The model under review builds one solid part; all positions refer to its coordinate system, in mm. A direction names the side the tool comes from. Give positions to 0.01 mm unless a question says otherwise; leave off trailing zeros. Order: outer loops, then holes, each group sorted by start corner. A loop starts at its lowest first (then second) coordinate and runs counter-clockwise, first axis right, second up.
```python
from build123d import *

# Parameters (mm, degrees)
SKETCH1_W               = 27
SKETCH1_H               = 129
BOSS_EXTRUDE1_DEPTH     = 1.5
FILLET1_R               = 3
SKETCH3_W               = 6
SKETCH3_H               = 3
CUT_EXTRUDE2_DEPTH      = 2.5
CUT_EXTRUDE2_DEPTH_BACK = 2.5
CUT_EXTRUDE4_DEPTH      = 2.5
CUT_EXTRUDE4_DEPTH_BACK = 2.5
FILLET2_R               = 3
FILLET2_2_R             = 1.5
CUT_EXTRUDE3_DEPTH      = 5
SKETCH2_W               = 3
SKETCH2_H               = 35
CUT_EXTRUDE1_DEPTH      = 2.5000001
CUT_EXTRUDE1_DEPTH_BACK = 2.5000001


with BuildPart() as part:
    # Sketch1 → Boss-Extrude1 (new body, symmetric)
    with BuildSketch(Plane(origin=(0, 0, 0), x_dir=(1, 0, 0), z_dir=(0, 1, 0))):
        Rectangle(SKETCH1_W, SKETCH1_H)
    extrude(amount=BOSS_EXTRUDE1_DEPTH, both=True)

    # Fillet1
    fillet1_edges = [part.edges().sort_by_distance(p)[0] for p in [
        (-13.5, 0, -64.5),
        (13.5, 0, -64.5),
    ]]
    fillet(fillet1_edges, radius=FILLET1_R)

    # Sketch3 → Cut-Extrude2 (cut, two sides)
    with BuildSketch(Plane(origin=(0, 0, 0), x_dir=(1, 0, 0), z_dir=(0, 1, 0))) as cut_extrude2_sk:
        with Locations((0, 63)):
            Rectangle(SKETCH3_W, SKETCH3_H)
    extrude(amount=CUT_EXTRUDE2_DEPTH, mode=Mode.SUBTRACT)
    extrude(cut_extrude2_sk.sketch, amount=-CUT_EXTRUDE2_DEPTH_BACK, mode=Mode.SUBTRACT)

    # Sketch5 → Cut-Extrude4 (cut, two sides)
    with BuildSketch(Plane(origin=(0, 0, 0), x_dir=(1, 0, 0), z_dir=(0, 1, 0))) as cut_extrude4_sk:
        with BuildLine():
            Line((-13.5, -52.5), (-13, -52.5))
            ThreePointArc((-13, -52.5), (-7.343145751, -54.843145751), (-5, -60.5))
            Line((-5, -60.5), (-5, -64.5))
            Line((-5, -64.5), (-13.5, -64.5))
            Line((-13.5, -64.5), (-13.5, -52.5))
        make_face()
        with BuildLine():
            Line((5, -60.5), (5, -64.5))
            Line((5, -64.5), (13.5, -64.5))
            Line((13.5, -64.5), (13.5, -52.5))
            Line((13.5, -52.5), (13, -52.5))
            ThreePointArc((13, -52.5), (7.343145751, -54.843145751), (5, -60.5))
        make_face()
    extrude(amount=CUT_EXTRUDE4_DEPTH, mode=Mode.SUBTRACT)
    extrude(cut_extrude4_sk.sketch, amount=-CUT_EXTRUDE4_DEPTH_BACK, mode=Mode.SUBTRACT)

    # Fillet2
    fillet2_edges = [part.edges().sort_by_distance(p)[0] for p in [
        (-13.5, 0, 52.5),
        (13.5, 0, 52.5),
    ]]
    fillet(fillet2_edges, radius=FILLET2_R)

    # Fillet2 2
    fillet2_2_edges = [part.edges().sort_by_distance(p)[0] for p in [
        (-5, 0, 64.5),
        (5, 0, 64.5),
    ]]
    fillet(fillet2_2_edges, radius=FILLET2_2_R)

    # Sketch4 → Cut-Extrude3 (cut, symmetric)
    with BuildSketch(Plane(origin=(0, 0, 0), x_dir=(1, 0, 0), z_dir=(0, 1, 0))):
        Polygon((0, -59.643928679), (2.165063509, -55.893928679), (-2.165063509, -55.893928679), align=None)
    extrude(amount=CUT_EXTRUDE3_DEPTH, both=True, mode=Mode.SUBTRACT)

    # Sketch2 → Cut-Extrude1 (cut, two sides)
    with BuildSketch(Plane(origin=(0, 0, 0), x_dir=(1, 0, 0), z_dir=(0, 1, 0))) as cut_extrude1_sk:
        with Locations((-9, 33.895)):
            Rectangle(SKETCH2_W, SKETCH2_H)
        with Locations((9, 33.895)):
            Rectangle(SKETCH2_W, SKETCH2_H)
        with Locations((9, -22.105)):
            Rectangle(SKETCH2_W, SKETCH2_H)
        with Locations((-9, -22.105)):
            Rectangle(SKETCH2_W, SKETCH2_H)
    extrude(amount=CUT_EXTRUDE1_DEPTH, mode=Mode.SUBTRACT)
    extrude(cut_extrude1_sk.sketch, amount=-CUT_EXTRUDE1_DEPTH_BACK, mode=Mode.SUBTRACT)


solid = part.part
```
Item 1: Draft analysis for pull direction Z (two halves, no side actions). For faces 1 (the cylindrical face through (6.78, -0.02, 55.47)), 2 (the flat face through (-10.5, 0, -34)), 3 (the flat face through (-13.5, 0, -5)), 4 (the cylindrical face through (12.64, -0.02, -63.6)), state which applies: released by +Z, released by -Z, zero draft, split by the parting line, or undercut.
Values found:
face 1: released by +Z
face 2: undercut
face 3: zero draft
face 4: released by -Z
Item 2: For faces 5 (the flat face through (-9, 0, 39.605)), 6 (the flat face through (5, 0, 62)), 7 (the flat face through (-5, 0, 62)), 8 (the flat face through (0, 0, -61.5)), list the 3-axis set-ups (+Z, -Z, +X, -X, +Y, -Y) from which the entire face can be reached by the end or side of a thin tool; tool diameter is ignored.
Values found:
face 5: +Y, -Y
face 6: +Z, +X, +Y, -Y
face 7: +Z, -X, +Y, -Y
face 8: -Z, +Y, -Y
Item 3: Take a section at A-A (z = 13). Give the boundary of the cut face in (x, y), and give its area (3 significant figures).
Values found:
outline: (-13.5, -1.5) - (-10.5, -1.5) - (-10.5, 1.5) - (-13.5, 1.5) - close; (-7.5, -1.5) - (7.5, -1.5) - (7.5, 1.5) - (-7.5, 1.5) - close; (10.5, -1.5) - (13.5, -1.5) - (13.5, 1.5) - (10.5, 1.5) - close
area: 63.0 mm2
Item 4: Clearance check with flat-ended pins moving along their axes: pin 1 Ø0.9 at (x, y) = (-0.5, 0.5) entering from -Z; pin 2 Ø1.5 at (x, y) = (8.5, 0.5) entering from +Z; pin 3 Ø1.5 at (x, y) = (-9.5, 0.5) entering from +Z. State where each tip first meets the part, or that it passes through.
Values found:
pin 1: stops at z = -61.5
pin 2: stops at z = 54.46
pin 3: stops at z = 53.72
Item 5: Take a section at B-B (x = -9). Give the boundary of the cut face in (y, z) (3 decimals).
Values found:
outline: (-1.5, -64.5) - (1.5, -64.5) - (1.5, -51.395) - (-1.5, -51.395) - close; (-1.5, -16.395) - (1.5, -16.395) - (1.5, 4.605) - (-1.5, 4.605) - close; (-1.5, 39.605) - (1.5, 39.605) - (1.5, 53.572) - (-1.5, 53.572) - close
Item 6: For line 1 (X direction, y = -0.75, z = -49); line 2 (Z direction, x = -10, y = 0.15) (3 decimals); line 3 (Z direction, x = 1.75, y = -0.9), list the stretches that pass through material, from the lowest coordinate up.
Values found:
line 1: x = -13.5 to -10.5, -7.5 to 7.5, 10.5 to 13.5
line 2: z = -64.5 to -51.395, -16.395 to 4.605, 39.605 to 53.084
line 3: z = -61.5 to 55.89, 56.61 to 64.5
Item 7: Take a section at C-C (y = 0.8). Give the number of separate pieces and of enclosed holes in the cut face, and give its area (3 significant figures).
Values found:
separate pieces: 1
enclosed holes: 5
area: 2,850 mm2
Item 8: Take a section at D-D (x = 6.25). Give the boundary of the cut face in (y, z), and give its area (3 significant figures).
Values found:
outline: (-1.5, -64.5) - (1.5, -64.5) - (1.5, 56.21) - (-1.5, 56.21) - close
area: 362 mm2
